Geometry: final body of the model. Coordinates: model frame, mm. A direction names the side the tool comes from. Round coordinates to 2 decimals unless told otherwise and drop trailing zeros. Write each loop counter-clockwise with the first axis right and the second up, starting at its lowest first coordinate (ties: lowest second). Pieces come first, ordered by that corner, then holes. Notation, with made-up numbers: (-14, 37) - (7, 37) arc R21 ccw to (7, 74) - close; hole circle Ø3 at (-16, 25). An arc over 180 degrees is marked (long way). Use a Markdown table: item, result. Add a question column.
Autodesk Inventor part; units mm, degrees
ref_plane "YZ Plane" through (0, 0, 0) normal (1, 0, 0) x (0, 1, 0)
ref_plane "XZ Plane" through (0, 0, 0) normal (0, 1, 0) x (-1, 0, 0)
ref_plane "XY Plane" through (0, 0, 0) normal (0, 0, 1) x (1, 0, 0)
sketch "Sketch1" plane through (0, 0, 0) normal (0, 1, 0) x (-1, 0, 0)
  line L0 (0, 0) -> (0, 152.4)
  line L1 (0, 152.4) -> (152.4, 152.4)
  line L2 (152.4, 152.4) -> (152.4, -152.4)
  line L3 (152.4, -152.4) -> (-152.4, -152.4)
  line L4 (-152.4, -152.4) -> (-152.4, 152.4)
  line L5 (-152.4, 152.4) -> (0, 152.4)
  dimension "d0" = 152.4
  dimension "d1" = 152.4
  dimension "d2" = 304.8
  dimension "d3" = 90
  dimension "d4" = 304.8
extrude "Extrusion1" add sketch "Sketch1" along normal blind 12.7
sketch "Sketch2" plane through (0, 12.7, 0) normal (0, 1, 0) x (1, 0, 0)
  line L0 (-152.4, -152.4) -> (152.4, -152.4)
  line L1 (-152.4, -152.4) -> (-152.4, -139.7)
  line L2 (-152.4, 152.4) -> (-152.4, -152.4)
  line L3 (-152.4, -139.7) -> (152.4, -139.7)
  line L4 (152.4, -152.4) -> (152.4, 152.4)
  line L5 (152.4, -139.7) -> (139.7, -139.7)
  line L6 (139.7, -139.7) -> (139.7, 139.7)
  line L7 (139.7, 139.7) -> (-139.7, 139.7)
  line L8 (-139.7, 139.7) -> (-139.7, -139.7)
  line L9 (152.4, 152.4) -> (-152.4, 152.4)
  point P0 (0, 0)
  dimension "d7" = 12.7
  dimension "d8" = 304.8
  dimension "d9" = 12.7
  dimension "d10" = 279.4
  dimension "d11" = 279.4
  dimension "d12" = 90
  dimension "d13" = 279.4
extrude "Extrusion2" add sketch "Sketch2" along normal blind 88.9 contours L1 L3 L4 L0 | L2 L9 L4 L3 L6 L7 L8
properties part number "Box with dimensions"
1) Draft query along X for faces 1 (the flat face through (-2, 50, -152.4)), 2 (the flat face through (2, 12.7, 2)), 3 (the flat face through (-152.4, 50, 2)). Return one class per face: released by +X, released by -X, zero draft, split by the parting line, or undercut.
2) Set-up query: faces 4 (the flat face through (152.4, 50, -2)), 5 (the flat face through (2, 57, -139.7)). Return all of +Z, -Z, +X, -X, +Y, -Y with unobstructed straight access to the full face (end or side cutting, diameter ignored); none if empty.
3) Material intervals for L1, parallel to Z at x = -3, y = 48; L2, parallel to Y at x = 99, z = -88, sorted ascending. Write a range as from..to.
4) Section A-A, the plane z = 107. Return the cut outline in (x, y).
5) Section C-C, the plane x = -82. Return the cut outline in (y, z).
6) Pin query (flat end, axial travel): P1, Ø8, axis at x = -23.5, z = 40, coming from the +Y side. Return the tip coordinate at first contact, or that it passes through.
7) Section B-B, the plane y = 67. Return the cut outline in (x, z).
Output values:
| question | item | result |
|---|---|---|
| 1 | face 1 | zero draft |
| 1 | face 2 | undercut |
| 1 | face 3 | released by -X |
| 2 | face 4 | +Z, -Z, +X, +Y, -Y |
| 2 | face 5 | +Y |
| 3 | L1 | z = -152.4..-139.7, 139.7..152.4 |
| 3 | L2 | y = 0..12.7 |
| 4 | outline | (-152.4, 0) - (152.4, 0) - (152.4, 101.6) - (139.7, 101.6) - (139.7, 12.7) - (-139.7, 12.7) - (-139.7, 101.6) - (-152.4, 101.6) - close |
| 5 | outline | (0, -152.4) - (101.6, -152.4) - (101.6, -139.7) - (12.7, -139.7) - (12.7, 139.7) - (101.6, 139.7) - (101.6, 152.4) - (0, 152.4) - close |
| 6 | P1 | stops at y = 12.7 |
| 7 | outline | (-152.4, -152.4) - (152.4, -152.4) - (152.4, 152.4) - (-152.4, 152.4) - close; hole (-139.7, -139.7) - (139.7, -139.7) - (139.7, 139.7) - (-139.7, 139.7) - close |
